```python
from build123d import *

# Parameters (mm, degrees)
SKETCH1_W               = 30
SKETCH1_H               = 15
BOSS_EXTRUDE1_DEPTH     = 180
SHELL2_T                = 2
SKETCH3_R               = 2.5
CUT_EXTRUDE3_DEPTH      = 50
MIRROR3_COPY_1_SKETCH_R = 2.5
MIRROR3_COPY_1_DEPTH    = 50
SKETCH7_W               = 34
SKETCH7_H               = 17
BOSS_EXTRUDE5_DEPTH     = 10
SKETCH12_R              = 1.5
CUT_EXTRUDE5_DEPTH      = 193.985103052
SKETCH13_R              = 1.5
CUT_EXTRUDE6_DEPTH      = 193.985103052


with BuildPart() as part:
    # Sketch1 → Boss-Extrude1 (new body)
    with BuildSketch(Plane.XY):
        Rectangle(SKETCH1_W, SKETCH1_H)
    extrude(amount=BOSS_EXTRUDE1_DEPTH)

    # Shell2
    shell2_openings = [part.faces().sort_by_distance(p)[0] for p in [
        (0, 7.5, 90),
        (0, 0, 0),
    ]]
    offset(amount=SHELL2_T, openings=shell2_openings, kind=Kind.INTERSECTION)

    # Sketch3 → Cut-Extrude3 (cut)
    with BuildSketch(Plane(origin=(15, 0, 0), x_dir=(0, 0, -1), z_dir=(1, 0, 0))):
        with Locations((-4.245349373, 0)):
            Circle(SKETCH3_R)
    cut_extrude3 = extrude(amount=-CUT_EXTRUDE3_DEPTH, mode=Mode.SUBTRACT)

    # Mirror1: Cut-Extrude3 across plane
    add(cut_extrude3.mirror(Plane.XY.offset(40)), mode=Mode.SUBTRACT)

    # Mirror3: Cut-Extrude3 across plane
    add(cut_extrude3.mirror(Plane(origin=(0, 0, 0), x_dir=(0, 0, 1), z_dir=(1, 0, 0))), mode=Mode.SUBTRACT)

    # Mirror3 copy 1 sketch → Mirror3 copy 1 (cut)
    with BuildSketch(Plane(origin=(-15, 0, 80), x_dir=(0, 0, 1), z_dir=(-1, 0, 0))):
        with Locations((-4.245349373, 0)):
            Circle(MIRROR3_COPY_1_SKETCH_R)
    extrude(amount=-MIRROR3_COPY_1_DEPTH, mode=Mode.SUBTRACT)

    # Sketch7 → Boss-Extrude5 (add)
    with BuildSketch(Plane.XY.offset(182)):
        with Locations((0, -1)):
            Rectangle(SKETCH7_W, SKETCH7_H)
    extrude(amount=BOSS_EXTRUDE5_DEPTH)

    # Sketch12 → Cut-Extrude5 (cut, through all)
    with BuildSketch(Plane.XY.offset(192)):
        with Locations((-8, 2.5)):
            Circle(SKETCH12_R)
        with Locations((-8, -5.054330526)):
            Circle(SKETCH12_R)
        with Locations((8, 2.5)):
            Circle(SKETCH12_R)
    extrude(amount=-CUT_EXTRUDE5_DEPTH, mode=Mode.SUBTRACT)

    # Sketch13 → Cut-Extrude6 (cut, through all)
    with BuildSketch(Plane.XY.offset(192)):
        with Locations((8, -5)):
            Circle(SKETCH13_R)
    extrude(amount=-CUT_EXTRUDE6_DEPTH, mode=Mode.SUBTRACT)


solid = part.part
```
Build history of the part. All positions in model axes, mm. A direction names the side the tool comes from. Give positions to 0.01 mm unless a question says otherwise; leave off trailing zeros. Loops run counter-clockwise (first coordinate to the right, second up) from the corner with the lowest first, then second, coordinate; pieces in that order, holes last.
1) Band-saw the part on B-B on x = -4.5. List the corners of the cut face in (y, z), then the cut area to 3 significant figures.
Values follow:
outline: (-9.5, 0) - (-7.5, 0) - (-7.5, 180) - (7.5, 180) - (7.5, 192) - (-9.5, 192) - close
area: 564 mm2
2) Probe line 1 along Y through (x, z) = (8, 183.75); line 2 along Y through (x, z) = (-8, 183.25); line 3 along X through (y, z) = (6, 140). List the from-to ranges inside material, lowest first.
Values follow:
line 1: y = -9.5 to -6.5, -3.5 to 1, 4 to 7.5
line 2: y = -9.5 to -6.55, -3.55 to 1, 4 to 7.5
line 3: x = -17 to -15, 15 to 17
3) 3-axis set-ups, long thin cutter, end or side, ignore diameter. For faces 1 (the face through (0, 0, 180)), 2 (the face through (1, -8, 0)): which of +Z, -Z, +X, -X, +Y, -Y reach the whole face in a straight line?
Values follow:
face 1: -Z, +Y
face 2: -Z, +X, -X, +Y, -Y
4) Drop flat-ended pins along their axis: P1, Ø3, axis at y = 0, z = 75.75, coming from the -X side; P2, Ø2, axis at x = -2.5, y = 0, coming from the -Z side; P3, Ø8, axis at y = 0, z = 4.25, coming from the -X side; P4, Ø1.5, axis at x = -10, z = 20.5, coming from the +Y side. Give the stop position or say it passes through.
Values follow:
P1: passes through
P2: stops at z = 180
P3: stops at x = -17
P4: stops at y = -7.5
5) Two-plate mould, pull along X, no slides. Class faces 3 (the face through (-17, -1, 95)), 4 (the face through (-15.2, 7.5, 124)), 5 (the face through (-15, 0, 89)): released by +X, released by -X, zero draft, split by the parting line, or undercut.
Values follow:
face 3: released by -X
face 4: zero draft
face 5: undercut
6) Band-saw the part on A-A on z = 98.5. List the corners of the cut face in (x, y), then the cut area to 3 significant figures.
Values follow:
outline: (-17, -9.5) - (17, -9.5) - (17, 7.5) - (15, 7.5) - (15, -7.5) - (-15, -7.5) - (-15, 7.5) - (-17, 7.5) - close
area: 128 mm2
